```python
from build123d import *

# Parameters (mm, degrees)
SKETCH1_W           = 42
SKETCH1_H           = 42
BOSS_EXTRUDE1_DEPTH = 8
SKETCH2_R           = 1.6
SKETCH2_R_2         = 7.5
CUT_EXTRUDE1_DEPTH  = 9
CHAMFER1_SIZE       = 3


with BuildPart() as part:
    # Sketch1 → Boss-Extrude1 (new body)
    with BuildSketch(Plane.XY):
        with Locations((21, 21)):
            Rectangle(SKETCH1_W, SKETCH1_H)
    extrude(amount=BOSS_EXTRUDE1_DEPTH)

    # Sketch2 → Cut-Extrude1 (cut)
    with BuildSketch(Plane.XY.offset(8)):
        with Locations((36.5, 5.5)):
            Circle(SKETCH2_R)
        with Locations((5.5, 5.5)):
            Circle(SKETCH2_R)
        with Locations((21, 21)):
            Circle(SKETCH2_R_2)
    extrude(amount=-CUT_EXTRUDE1_DEPTH, mode=Mode.SUBTRACT)

    # Chamfer1
    chamfer1_edges = [part.edges().sort_by_distance(p)[0] for p in [
        (0, 42, 4),
        (42, 42, 4),
        (42, 0, 4),
        (0, 0, 4),
    ]]
    chamfer(chamfer1_edges, length=CHAMFER1_SIZE)


solid = part.part
```
Geometry: final body of the model. Coordinates: model frame, mm. Coordinates: 2 decimals unless noted, no trailing zeros. Loops run counter-clockwise (first coordinate to the right, second up) from the corner with the lowest first, then second, coordinate; pieces in that order, holes last. Notation, with made-up numbers: M 68,25.5 L 105,25.5 A17 ccw 105,48.5 Z; hole C 41,79.25 d4. An arc over 180 degrees is marked long. Put each result on its own line as item: value.
(1) Cut plane B-B on y = 5.5. Return the cut outline in (x, z), then the cut area to 3 significant figures.
Answer sheet:
outline: M 0,0 L 3.9,0 L 3.9,8 L 0,8 Z; M 7.1,0 L 34.9,0 L 34.9,8 L 7.1,8 Z; M 38.1,0 L 42,0 L 42,8 L 38.1,8 Z
area: 285 mm^2
(2) Cut plane D-D on z = 5.5. Return the cut outline in (x, y).
Answer sheet:
outline: M 0,3 L 3,0 L 39,0 L 42,3 L 42,39 L 39,42 L 3,42 L 0,39 Z; hole C 5.5,5.5 d3.2; hole C 21,21 d15; hole C 36.5,5.5 d3.2
(3) Cut plane C-C on x = 5.5. Return the cut outline in (y, z), then the cut area to 3 significant figures.
Answer sheet:
outline: M 0,0 L 3.9,0 L 3.9,8 L 0,8 Z; M 7.1,0 L 42,0 L 42,8 L 7.1,8 Z
area: 310 mm^2
(4) Draft query along Y for faces 1 (the face through (30, 21, 0)), 2 (the face through (41, 40, 4)), 3 (the face through (15.5, 26.1, 4.1)), 4 (the face through (41, 2, 4)). Return one class per face: pulls with the +Y half, pulls with the -Y half, needs draft (parallel to the pull), parting line crosses it, or undercut.
Answer sheet:
face 1: needs draft
face 2: pulls with the +Y half
face 3: undercut
face 4: pulls with the -Y half
(5) Material intervals for probe 1 along Y at (x, z) = (36.5, 4.5); probe 2 along Y at (x, z) = (23.5, 1.25); probe 3 along X at (y, z) = (22.5, 5.5), sorted ascending.
Answer sheet:
probe 1: y = 0 to 3.9, 7.1 to 42
probe 2: y = 0 to 13.93, 28.07 to 42
probe 3: x = 0 to 13.65, 28.35 to 42
(6) First-contact query: pin 1 (2 mm diameter, centred on x = 14.5, y = 37.5, fed in from -Z). Flat tip, straight axial feed; report the tip coordinate or a pass-through.
Answer sheet:
pin 1: stops at z = 0
(7) Cut plane A-A on y = 21. Return the cut outline in (x, z), then the cut area to 3 significant figures.
Answer sheet:
outline: M 0,0 L 13.5,0 L 13.5,8 L 0,8 Z; M 28.5,0 L 42,0 L 42,8 L 28.5,8 Z
area: 216 mm^2
